Source: three-view drawing plus pictorial views. Frame: mm from the lowest corner of the part. Round coordinates to 2 decimals unless told otherwise and drop trailing zeros. Loops run counter-clockwise (first coordinate to the right, second up) from the corner with the lowest first, then second, coordinate; pieces in that order, holes last. Notation, with made-up numbers: (84, 75.25) -> (111, 75.25) arc R30 ccw to (111, 107.25) -> close; hole circle Ø7 at (30, -8.75). An arc over 180 degrees is marked (long way). Answer as a JSON object with one key per item and string values. Group by question number.
Item 1: Section query B-B on x = 112.5. Return loops of the section in (y, z), and give its area (3 significant figures).
Item 2: Section query A-A on z = 62.5. Return loops of the section in (x, y), and give its area (3 significant figures).
Item 3: Section query C-C on z = 112.5. Return loops of the section in (x, y), and give its area (3 significant figures).
Item 4: Material intervals for line 1 (X direction, y = 2.65, z = 112.5); line 2 (Z direction, x = 111, y = 3.15) (1 decimal), sorted ascending. Write a range as [from, to].
Item 5: Section query D-D on y = 1. Count the separate pieces of the cut face and the enclosed holes in it, and give its area (3 significant figures).
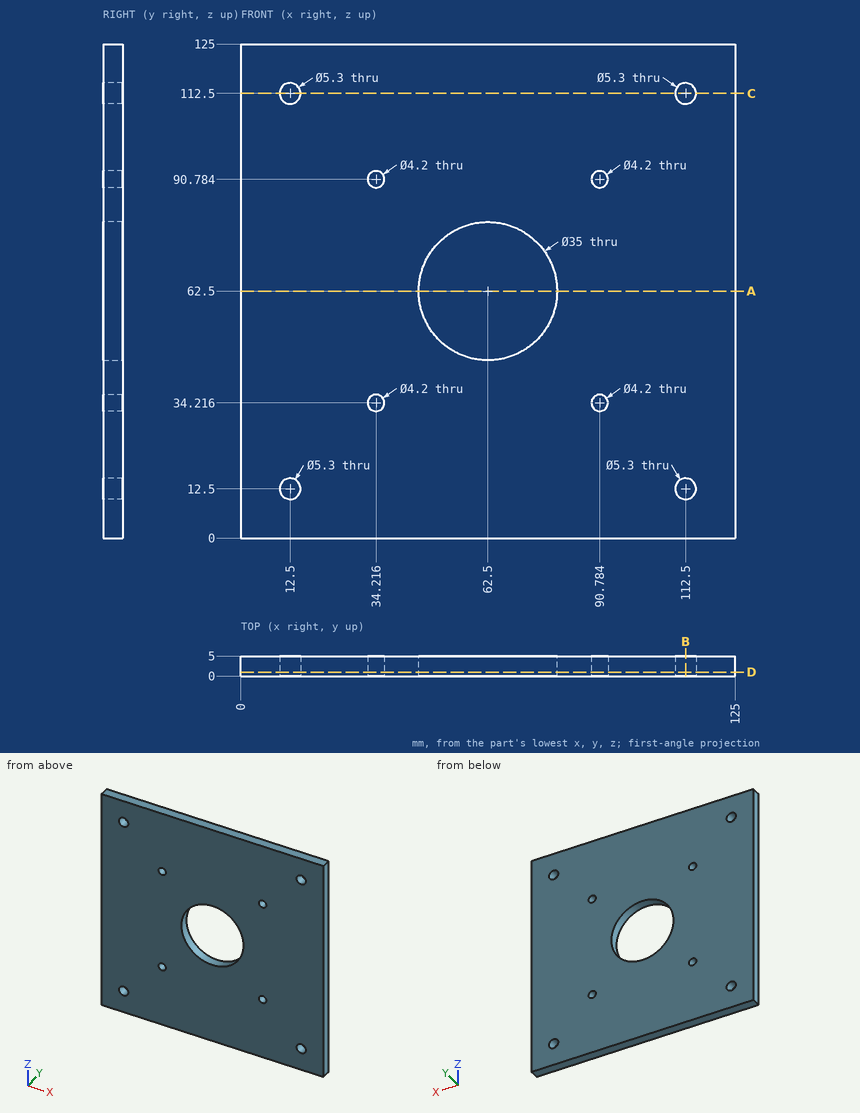
Solved:
{
 "1": {"outline": "(0, 0) -> (5, 0) -> (5, 9.85) -> (0, 9.85) -> close; (0, 15.15) -> (5, 15.15) -> (5, 109.85) -> (0, 109.85) -> close; (0, 115.15) -> (5, 115.15) -> (5, 125) -> (0, 125) -> close", "area": "572 mm²"},
 "2": {"outline": "(0, 0) -> (45, 0) -> (45, 5) -> (0, 5) -> close; (80, 0) -> (125, 0) -> (125, 5) -> (80, 5) -> close", "area": "450 mm²"},
 "3": {"outline": "(0, 0) -> (9.85, 0) -> (9.85, 5) -> (0, 5) -> close; (15.15, 0) -> (109.85, 0) -> (109.85, 5) -> (15.15, 5) -> close; (115.15, 0) -> (125, 0) -> (125, 5) -> (115.15, 5) -> close", "area": "572 mm²"},
 "4": {"line 1": "[0, 9.85], [15.15, 109.85], [115.15, 125]", "line 2": "[0, 10.3], [14.7, 110.3], [114.7, 125]"},
 "5": {"separate pieces": "1", "enclosed holes": "9", "area": "14,500 mm²"}
}
